from build123d import *

# Parameters (mm, degrees)
SKETCH1_R               = 27
BOSS_EXTRUDE1_DEPTH     = 63.5
SKETCH2_R               = 25
BOSS_EXTRUDE2_DEPTH     = 127
CUT_EXTRUDE1_DEPTH      = 195.289088731
CUT_EXTRUDE1_DEPTH_BACK = 195.289088731


with BuildPart() as part:
    # Sketch1 → Boss-Extrude1 (new body)
    with BuildSketch(Plane.XY):
        Circle(SKETCH1_R)
    extrude(amount=BOSS_EXTRUDE1_DEPTH)

    # Sketch2 → Boss-Extrude2 (add)
    with BuildSketch(Plane.XY.offset(63.5)):
        Circle(SKETCH2_R)
    extrude(amount=BOSS_EXTRUDE2_DEPTH)

    # Sketch4 → Cut-Extrude1 (cut, two sides: drawn at the far end of the back side and taken through both)
    with BuildSketch(Plane(origin=(0, 0, 0), x_dir=(1, 0, 0), z_dir=(0, 1, 0)).offset(-CUT_EXTRUDE1_DEPTH_BACK)):
        Polygon((-25, -72.711167147), (-23.8, -74.5), (-23.8, -105.5), (-25, -107.288832853), align=None)
        Polygon((-27.757940887, -16.532917761), (-27.757940887, -43.467082239), (-23.5, -40.5), (-23.5, -19.5), align=None)
        Polygon((23.8, -74.5), (23.8, -105.5), (25, -107.288832853), (25, -72.711167147), align=None)
        Polygon((27.757940887, -16.532917761), (27.757940887, -43.467082239), (23.5, -40.5), (23.5, -19.5), align=None)
    extrude(amount=CUT_EXTRUDE1_DEPTH + CUT_EXTRUDE1_DEPTH_BACK, mode=Mode.SUBTRACT)


solid = part.part
Could you check a few things on this model? Use its own coordinates, in mm. A direction names the side the tool comes from. Coordinates: 2 decimals unless noted, no trailing zeros. Write each loop counter-clockwise with the first axis right and the second up, starting at its lowest first coordinate (ties: lowest second). Pieces come first, ordered by that corner, then holes. Notation, with made-up numbers: (-18.5, 63) - (18.5, 63) arc R22 cw to (18.5, 93) - close; hole circle Ø3 at (-13, 73). An arc over 180 degrees is marked (long way). Write item = value, one per line.
1) Suppose I cut it at A-A on x = 0. Please give me the cut outline in (y, z), plus the area to 3 significant figures.
Result set:
outline = (-27, 0) - (27, 0) - (27, 63.5) - (25, 63.5) - (25, 190.5) - (-25, 190.5) - (-25, 63.5) - (-27, 63.5) - close
area = 9,780 mm2
2) Please list where these lines run through material, in increasing order: line 1 (X direction, y = 3.5, z = 37.5); line 2 (X direction, y = 7.5, z = 87); line 3 (Y direction, x = 0, z = 171). Write a range as [from, to].
Result set:
line_1 = [-23.5, 23.5]
line_2 = [-23.8, 23.8]
line_3 = [-25, 25]
3) Suppose I cut it at C-C on z = 100.5. Please give me the cut outline in (x, y).
Result set:
outline = (-23.8, -7.65) arc R25 ccw to (23.8, -7.65) - (23.8, 7.65) arc R25 ccw to (-23.8, 7.65) - close
4) Suppose I cut it at D-D on x = -12.5. Please give me the cut outline in (y, z).
Result set:
outline = (-23.93, 0) - (23.93, 0) - (23.93, 63.5) - (21.65, 63.5) - (21.65, 190.5) - (-21.65, 190.5) - (-21.65, 63.5) - (-23.93, 63.5) - close
5) Suppose I cut it at B-B on y = 0. Please give me the cut outline in (x, z), plus the area to 3 significant figures.
Result set:
outline = (-27, 0) - (27, 0) - (27, 17.06) - (23.5, 19.5) - (23.5, 40.5) - (27, 42.94) - (27, 63.5) - (25, 63.5) - (25, 72.71) - (23.8, 74.5) - (23.8, 105.5) - (25, 107.29) - (25, 190.5) - (-25, 190.5) - (-25, 107.29) - (-23.8, 105.5) - (-23.8, 74.5) - (-25, 72.71) - (-25, 63.5) - (-27, 63.5) - (-27, 42.94) - (-23.5, 40.5) - (-23.5, 19.5) - (-27, 17.06) - close
area = 9,540 mm2
6) We'd pull the mould along Z, two halves only. Please class faces 1 (the flat face through (0, 0, 190.5)), 2 (the flat face through (-24.89, -0.19, 41.47)), 3 (the flat face through (0, 0, 0)): +Z half, -Z half, draft (parallel to the pull), parting line (faces both ways), or undercut.
Result set:
face_1 = +Z half
face_2 = undercut
face_3 = -Z half
7) Will these pins go through, and if not, where does the flat tip stop? pin 1 Ø6.5 at (y, z) = (-1.5, 25.5) entering from +X; pin 2 Ø8 at (x, z) = (-13, 98.5) entering from -Y; pin 3 Ø8 at (y, z) = (-11, 107.5) entering from +X.
Result set:
pin_1 = 23.5
pin_2 = -23.32
pin_3 = 24
8) For faces 4 (the cylindrical face through (-21.426, -16.429, 31.306)), 5 (the flat face through (24.837, -0.186, 18.569)), 6 (the cylindrical face through (11.5, -22.2, 126.1)), 7 (the flat face through (-23.8, 0, 90)), which set-ups out of +Z, -Z, +X, -X, +Y, -Y let a thin tool reach every point of the face, with its end or its side?
Result set:
face_4 = +Z, -Z
face_5 = +X, +Y, -Y
face_6 = +Z
face_7 = -X, +Y, -Y
